Input: part model. Units: mm. Frame: model coordinates. A direction names the side the tool comes from. Round coordinates to 2 decimals unless told otherwise and drop trailing zeros. Loops run counter-clockwise (first coordinate to the right, second up) from the corner with the lowest first, then second, coordinate; pieces in that order, holes last. Notation, with made-up numbers: (-19.5, 9.5) -> (-13.5, 9.5) arc R20 ccw to (-13.5, 17.5) -> close; hole circle Ø3 at (4, -8.75). An arc over 180 degrees is marked (long way). Answer as a JSON object with one key per item and string values.
```python
from build123d import *

# Parameters (mm, degrees)
ESBO_O1_R                = 2
RESSALTO_EXTRUS_O1_DEPTH = 2.5
ESBO_O1_3_R              = 1.25
RESSALTO_EXTRUS_O2_DEPTH = 7
RESSALTO_EXTRUS_O3_START = 2
ESBO_O1_4_R              = 1.25
RESSALTO_EXTRUS_O3_DEPTH = 2
ESBO_O2_W                = 2.5
ESBO_O2_H                = 5
RESSALTO_EXTRUS_O4_DEPTH = 1.5


with BuildPart() as part:
    # Esbo_o1 → Ressalto-extrus_o1 (new body)
    with BuildSketch(Plane(origin=(0, 0, 0), x_dir=(1, 0, 0), z_dir=(0, 1, 0))):
        with BuildLine():
            ThreePointArc((-10.1, 9), (-11.35, 10.25), (-12.6, 9))
            Line((-12.6, 9), (-12.6, 4))
            Line((-12.6, 4), (-1.904447094, -2.936508346))
            ThreePointArc((-1.904447094, -2.936508346), (0, -3.5), (1.904447094, -2.936508346))
            Line((1.904447094, -2.936508346), (12.6, 4))
            Line((12.6, 4), (12.6, 9))
            ThreePointArc((12.6, 9), (11.35, 10.25), (10.1, 9))
            Line((10.1, 9), (10.1, 5.954321796))
            Line((10.1, 5.954321796), (3.178453386, 1.465412595))
            ThreePointArc((3.178453386, 1.465412595), (0, 3.5), (-3.178453386, 1.465412595))
            Line((-3.178453386, 1.465412595), (-10.1, 5.954321796))
            Line((-10.1, 5.954321796), (-10.1, 9))
        make_face()
        with Locations(Location((0, 0, 0), (0, 0, 270))):
            Circle(ESBO_O1_R, mode=Mode.SUBTRACT)
    extrude(amount=-RESSALTO_EXTRUS_O1_DEPTH)

    # Esbo_o1_3 → Ressalto-extrus_o2 (add)
    with BuildSketch(Plane(origin=(0, 0, 0), x_dir=(1, 0, 0), z_dir=(0, 1, 0))):
        with BuildLine():
            Line((-10.1, 5.954321796), (-10.1, 9))
            ThreePointArc((-10.1, 9), (-11.35, 7.75), (-12.6, 9))
            Line((-12.6, 9), (-12.6, 4))
            Line((-12.6, 4), (-10.1, 4))
            Line((-10.1, 4), (-10.1, 5.954321796))
        make_face()
        with Locations((-11.35, 9)):
            Circle(ESBO_O1_3_R)
        with Locations((11.35, 9)):
            Circle(ESBO_O1_3_R)
        with BuildLine():
            Line((10.1, 9), (10.1, 5.954321796))
            Line((10.1, 5.954321796), (10.1, 4))
            Line((10.1, 4), (12.6, 4))
            Line((12.6, 4), (12.6, 9))
            ThreePointArc((12.6, 9), (11.35, 7.75), (10.1, 9))
        make_face()
    extrude(amount=-RESSALTO_EXTRUS_O2_DEPTH)

    # Esbo_o1_4 → Ressalto-extrus_o3 (add)
    with BuildSketch(Plane(origin=(0, 0, 0), x_dir=(1, 0, 0), z_dir=(0, 1, 0)).offset(RESSALTO_EXTRUS_O3_START)):
        with Locations(Location((-11.35, 9, 0), (0, 0, 270))):
            Circle(ESBO_O1_4_R)
        with Locations(Location((11.35, 9, 0), (0, 0, 270))):
            Circle(ESBO_O1_4_R)
    extrude(amount=-RESSALTO_EXTRUS_O3_DEPTH)

    # Esbo_o2 → Ressalto-extrus_o4 (add)
    with BuildSketch(Plane.XZ.offset(7)):
        with Locations((-11.35, -6.5)):
            Rectangle(ESBO_O2_W, ESBO_O2_H)
        with Locations((11.35, -6.5)):
            Rectangle(ESBO_O2_W, ESBO_O2_H)
    extrude(amount=RESSALTO_EXTRUS_O4_DEPTH)


solid = part.part
```
1) Draft query along X for faces 6 (the face through (-11, -8, -9)), 7 (the face through (6.688, -1.232, -3.741)), 8 (the face through (-7.33, -1.23, -0.58)), 9 (the face through (12.6, -4, -6)). Return one class per face: +X half, -X half, draft (parallel to the pull), parting line (faces both ways), or undercut.
Output:
{"face 6": "draft", "face 7": "undercut", "face 8": "-X half", "face 9": "+X half"}
2) Section C-C, the plane y = -1. Output: boundary loops of the cut face in (x, z).
Output:
{"outline": "(-12.6, -9) arc R1.25 ccw to (-10.1, -9) -> (-10.1, -5.95) -> (-3.18, -1.47) arc R3.5 ccw to (3.18, -1.47) -> (10.1, -5.95) -> (10.1, -9) arc R1.25 ccw to (12.6, -9) -> (12.6, -4) -> (1.9, 2.94) arc R3.5 ccw to (-1.9, 2.94) -> (-12.6, -4) -> close; hole circle Ø4 at (0, 0)"}
3) Section D-D, the plane x = 10.5. Output: boundary loops of the cut face in (y, z).
Output:
{"outline": "(-8.5, -9) -> (-7, -9) -> (-7, -9.92) -> (2, -9.92) -> (2, -8.08) -> (0, -8.08) -> (0, -2.64) -> (-2.5, -2.64) -> (-2.5, -4) -> (-8.5, -4) -> close"}
4) Contact query for flat-ended pins moving along their axis: P1, Ø2, axis at x = -9, z = -4.5, coming from the +Y side; P2, Ø3, axis at x = -11.5, y = -6.5, coming from the +Z side; P3, Ø0.8, axis at x = -11, y = -7.5, coming from the -Z side. Output: stop coordinate, or through.
Output:
{"P1": "stops at y = 0", "P2": "stops at z = -4", "P3": "stops at z = -9"}
5) Ray query, probe 1 along X at (y, z) = (-1.25, -2.75); probe 2 along X at (y, z) = (-6.75, -8); probe 3 along X at (y, z) = (-1.9, 0). Return the intervals inside material, ascending.
Output:
{"probe 1": "x = -10.67 to -5.16, -2.17 to 2.17, 5.16 to 10.67", "probe 2": "x = -12.6 to -10.1, 10.1 to 12.6", "probe 3": "x = -6.43 to -2, 2 to 6.43"}
6) Reachability of faces 1 (the face through (-2, -1, 0)), 2 (the face through (11, -5, -4)), 3 (the face through (7.2, -1.2, -0.5)), 4 (the face through (10.1, -4, -7)), 5 (the face through (11.3, -7, -9.5)) from +Z, -Z, +X, -X, +Y, -Y: full face, straight path, thin tool, end or side. Return the list, or none.
Output:
{"face 1": "+Y, -Y", "face 2": "+Z, +X, -X, -Y", "face 3": "+Z, +X, +Y, -Y", "face 4": "-Z, -Y", "face 5": "-Z, +X, -X, -Y"}
7) Section B-B, the plane x = 0. Output: boundary loops of the cut face in (y, z).
Output:
{"outline": "(-2.5, -3.5) -> (0, -3.5) -> (0, -2) -> (-2.5, -2) -> close; (-2.5, 2) -> (0, 2) -> (0, 3.5) -> (-2.5, 3.5) -> close"}
8) Section A-A, the plane y = -6.5. Output: boundary loops of the cut face in (x, z), plus the area to 3 significant figures.
Output:
{"outline": "(-12.6, -9) arc R1.25 ccw to (-10.1, -9) -> (-10.1, -4) -> (-12.6, -4) -> close; (10.1, -9) arc R1.25 ccw to (12.6, -9) -> (12.6, -4) -> (10.1, -4) -> close", "area": "29.9 mm^2"}
